Design review of the part shown in the three views and the two pictorial views. Dimensions are in mm from the part's minimum x, y and z. A direction names the side the tool comes from. Round coordinates to 2 decimals unless told otherwise and drop trailing zeros. Loops run counter-clockwise (first coordinate to the right, second up) from the corner with the lowest first, then second, coordinate; pieces in that order, holes last. Notation, with made-up numbers: (-19, 27) - (-1, 27) arc R13 cw to (-1, 44) - close; hole circle Ø3 at (41, 57.5). An arc over 180 degrees is marked (long way). Return JSON: item names as keys, results as strings. Group by question number.
(1) For the marked faces 1 and 2, list the 3-axis set-ups (+Z, -Z, +X, -X, +Y, -Y) from which the entire face can be reached by the end or side of a thin tool; tool diameter is ignored.
(2) We need section D-D, the plane z = 43.5. Write out the cut boundary in (x, y), and give its area (3 significant figures).
(3) We need section C-C, the plane x = 29.5. Write out the cut boundary in (y, z), and give its area (3 significant figures).
(4) We need section B-B, the plane z = 35. Write out the cut boundary in (x, y), and give its area (3 significant figures).
(5) We need section A-A, the plane y = 35. Write out the cut boundary in (x, z), and give its area (3 significant figures).
(6) Wall thickness on L1, parallel to X at y = 55.5, z = 41; L2, parallel to X at y = 47, z = 3; L3, parallel to Z at x = 20.5, y = 12: over which ranges is each line inside the solid? List them lowest first. Write a range as [from, to].
(7) Clearance check with flat-ended pins moving along their axes: pin 1 (6 mm diameter, centred on y = 49.5, z = 40.5, fed in from +X); pin 2 (2.5 mm diameter, centred on y = 13.79, z = 13.79, fed in from -X); pin 3 (4 mm diameter, centred on y = 56, z = 8, fed in from -X); pin 4 (3 mm diameter, centred on x = 17.5, y = 15, fed in from +Z) (1 decimal). State where each tip first meets the part, or that it passes through.
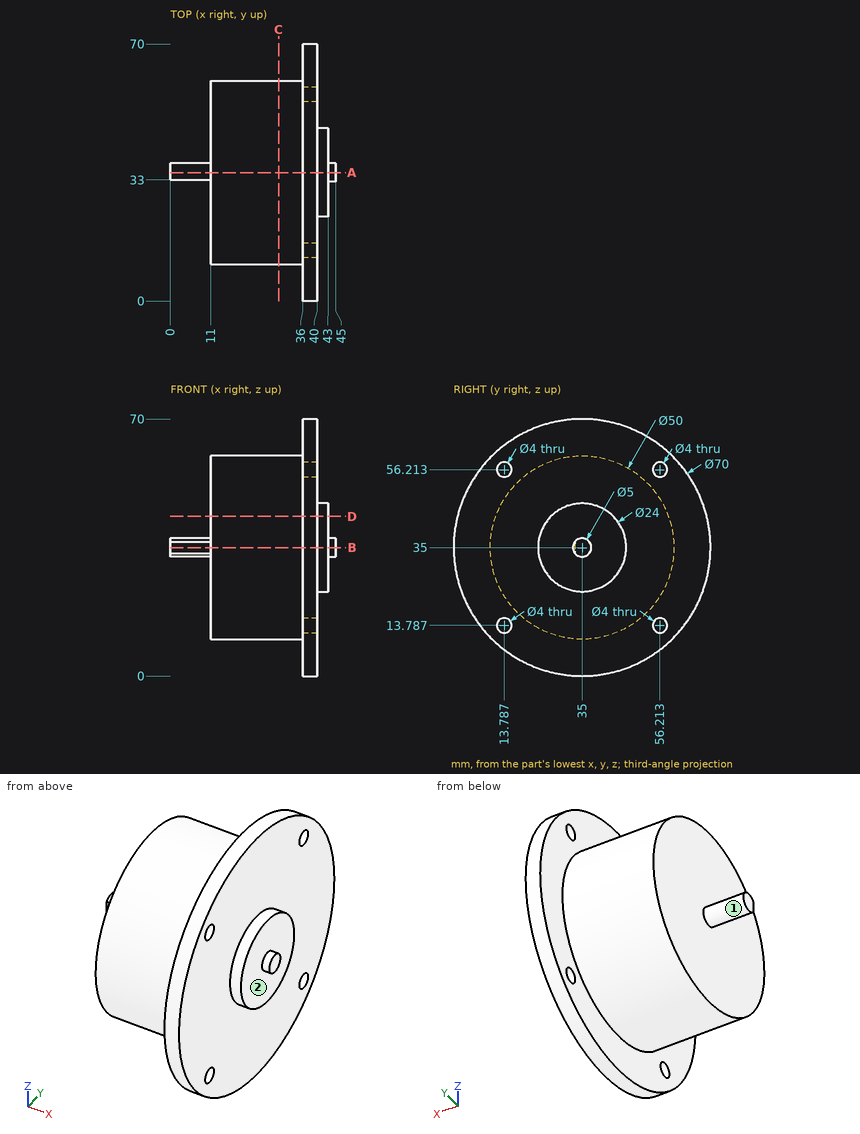
Solutions:
{
 "1": {"face 1": "-X", "face 2": "+X"},
 "2": {"outline": "(11, 11.49) - (36, 11.49) - (36, 1.05) - (40, 1.05) - (40, 26.53) - (43, 26.53) - (43, 43.47) - (40, 43.47) - (40, 68.95) - (36, 68.95) - (36, 58.51) - (11, 58.51) - close", "area": "1,500 mm^2"},
 "3": {"outline": "circle Ø50 at (35, 35)", "area": "1,960 mm^2"},
 "4": {"outline": "(0, 33) - (11, 33) - (11, 10) - (36, 10) - (36, 0) - (40, 0) - (40, 23) - (43, 23) - (43, 32.5) - (45, 32.5) - (45, 37.5) - (43, 37.5) - (43, 47) - (40, 47) - (40, 70) - (36, 70) - (36, 60) - (11, 60) - (11, 37.5) - (0, 37.5) - close", "area": "1,660 mm^2"},
 "5": {"outline": "(0, 32.5) - (11, 32.5) - (11, 10) - (36, 10) - (36, 0) - (40, 0) - (40, 23) - (43, 23) - (43, 32.5) - (45, 32.5) - (45, 37.5) - (43, 37.5) - (43, 47) - (40, 47) - (40, 70) - (36, 70) - (36, 60) - (11, 60) - (11, 37.5) - (0, 37.5) - close", "area": "1,670 mm^2"},
 "6": {"L1": "[11, 40]", "L2": "[36, 40]", "L3": "[25.2, 44.8]"},
 "7": {"pin 1": "x = 40", "pin 2": "through", "pin 3": "x = 36", "pin 4": "z = 51.8"}
}
